Geometry check sheet. Reference: the model listing, model coordinates, mm. Face numbers are marked on the shaded views. A direction names the side the tool comes from. Coordinates: 2 decimals unless noted, no trailing zeros. Order: outer loops, then holes, each group sorted by start corner. A loop starts at its lowest first (then second) coordinate and runs counter-clockwise, first axis right, second up. Notation, with made-up numbers: (25.5, 63) - (45.5, 63) arc R17 ccw to (45.5, 80) - close; hole circle Ø5 at (-37.75, -17.5). An arc over 180 degrees is marked (long way). Return JSON: item names as keys, results as strings. Group by question number.
Item 1: Section check B-B on z = -13. Enter the section's corners in (x, y), then the cut area to 3 significant figures.
Item 2: Tool access check on the marked faces 1 and 2. Record the directions out of +Z, -Z, +X, -X, +Y, -Y that give a thin tool (end or side, any length) a straight path to the whole face; none if there is none.
Item 3: Section check A-A on x = -19. Enter the section's corners in (y, z).
Item 4: Section check D-D on z = -53. Enter the section's corners in (x, y).
Item 5: Section check C-C on y = 16.25. Enter the section's corners in (x, z), then the cut area to 3 significant figures.
Item 6: Gauge pin test, flat ends, axial feed: pin 1 (1 mm diameter, centred on x = 3, y = 4, fed in from -Z); pin 2 (4.5 mm diameter, centred on x = 4, z = -32.5, fed in from +Y); pin 3 (6 mm diameter, centred on x = -1.5, y = 9, fed in from +Z); pin 4 (3 mm diameter, centred on y = 16, z = -41, fed in from +X). Record the tip position at first contact, or that the pin passes through.
Item 7: Scan lines: probe 1 along Z at (x, y) = (-19, 0.5); probe 2 along Y at (x, z) = (8, -28); probe 3 along X at (y, z) = (10, -34.5). Record each from-to range of solid material in increasing order.
Autodesk Inventor part; units mm, degrees
ref_plane "Work Plane1" through (-38, 20, -25) normal (0, 0, 1) x (1, 0, 0)
ref_plane "YZ Plane" through (0, 0, 0) normal (1, 0, 0) x (0, 1, 0)
ref_plane "XZ Plane" through (0, 0, 0) normal (0, 1, 0) x (-1, 0, 0)
sketch "Sketch1" plane through (0, 0, 0) normal (0, 1, 0) x (-1, 0, 0)
  line L0 (0, 0) -> (38, 0)
  line L1 (38, 0) -> (38, -50)
  line L2 (38, -50) -> (0, -50)
  line L3 (0, -50) -> (0, 0)
  dimension "d0" = 38
  dimension "d1" = 50
extrude "Extrusion1" add sketch "Sketch1" along normal blind 20
sketch "Sketch2" plane through (0, 0, 0) normal (0, -1, 0) x (1, 0, 0)
  line L0 (0, 0) -> (0, -50)
  line L1 (0, 0) -> (15, 0)
  line L2 (15, 0) -> (15, -50)
  line L3 (15, -50) -> (0, -50)
  line L4 (0, -50) -> (0, 0)
  dimension "d4" = 15
  dimension "d5" = 50
extrude "Extrusion2" add sketch "Sketch2" against normal blind 2
sketch "Sketch3" plane through (0, 0, 0) normal (0, -1, 0) x (1, 0, 0)
  line L0 (-38, 0) -> (0, 0)
  line L1 (-19, 0) -> (-19, 7)
  line L2 (-19, 0) -> (-19, 3)
  line L3 (-19, 0) -> (-10.5, 0)
  line L4 (-19, 0) -> (-27.5, 0)
  circle A0 centre (-19, 3) radius 1.5
  circle A1 centre (-19, 3) radius 4
  line L5 (-10.5, 0) -> (-17.4608, 6.692)
  line L6 (-27.5, 0) -> (-20.5392, 6.692)
  dimension "d10" = 8.5
  dimension "d11" = 8.5
  dimension "d12" = 3
  dimension "d18" = 3
  dimension "d19" = 8
extrude "Extrusion3" add sketch "Sketch3" against normal blind 2 contours L6 A1 L0 | A1 L6 L1 A0 L0 | L1 A0 A1 L5 L0 | A1 L5 L0
ref_plane "Work Plane1" through (-38, 20, -25) normal (0, 0, 1) x (1, 0, 0)
mirror "Mirror1" about plane through (-38, 20, -25) normal (0, 0, 1) of "Extrusion3"
properties part number "25W_1224_5V"
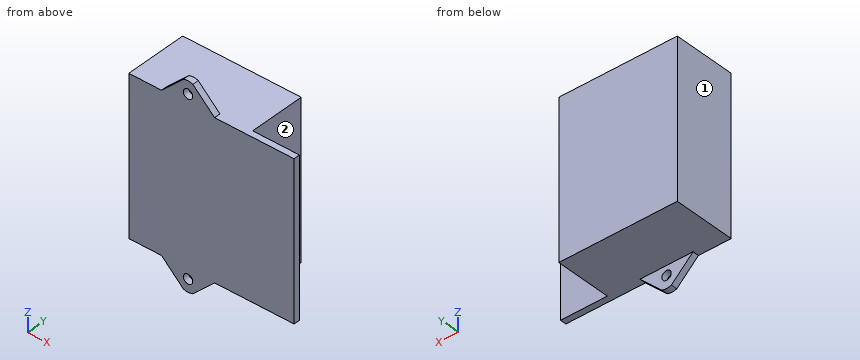
Computed:
{
 "1": {"outline": "(-38, 0) - (15, 0) - (15, 2) - (0, 2) - (0, 20) - (-38, 20) - close", "area": "790 mm²"},
 "2": {"face 1": "+Z, -Z, -X, +Y, -Y", "face 2": "+Z, -Z, +X, +Y"},
 "3": {"outline": "(0, -57) - (2, -57) - (2, -54.5) - (0, -54.5) - close; (0, -51.5) - (2, -51.5) - (2, -50) - (20, -50) - (20, 0) - (2, 0) - (2, 1.5) - (0, 1.5) - close; (0, 4.5) - (2, 4.5) - (2, 7) - (0, 7) - close"},
 "4": {"outline": "(-24.38, 0) - (-20.5, 0) - (-20.5, 2) - (-24.38, 2) - close; (-17.5, 0) - (-13.62, 0) - (-13.62, 2) - (-17.5, 2) - close"},
 "5": {"outline": "(-38, -50) - (0, -50) - (0, 0) - (-38, 0) - close", "area": "1,900 mm²"},
 "6": {"pin 1": "passes through", "pin 2": "stops at y = 2", "pin 3": "stops at z = 0", "pin 4": "stops at x = 0"},
 "7": {"probe 1": "z = -57 to -54.5, -51.5 to 1.5, 4.5 to 7", "probe 2": "y = 0 to 2", "probe 3": "x = -38 to 0"}
}
